from build123d import *

# Parameters (mm, degrees)
BOSS_EXTRUDE1_DEPTH     = 3
SKETCH2_R               = 4
SKETCH2_R_2             = 1.5
BOSS_EXTRUDE2_DEPTH     = 16
BOSS_EXTRUDE4_DEPTH     = 34
SKETCH6_R               = 5
SKETCH6_W               = 13
SKETCH6_H               = 12.705942109
SKETCH6_W_2             = 20
SKETCH6_H_2             = 11.5
CUT_EXTRUDE1_DEPTH      = 10
CUT_EXTRUDE1_DEPTH_BACK = 5
SKETCH9_R               = 12.7
CUT_EXTRUDE3_DEPTH      = 8
SKETCH10_R              = 1
CUT_EXTRUDE4_DEPTH      = 10
FILLET1_R               = 1
SKETCH11_R              = 1.62
SKETCH11_W              = 6.5
SKETCH11_H              = 17.5
CUT_EXTRUDE5_DEPTH      = 10


with BuildPart() as part:
    # Sketch1 → Boss-Extrude1 (new body)
    with BuildSketch(Plane(origin=(0, 0, 0), x_dir=(1, 0, 0), z_dir=(0, 1, 0))):
        with BuildLine():
            Line((-104.6543947, -23.181164953), (-24.598685103, -57.455675883))
            ThreePointArc((-24.598685103, -57.455675883), (62.5, 0), (-24.598685103, 57.455675883))
            Line((-24.598685103, 57.455675883), (-104.6543947, 23.181164953))
            ThreePointArc((-104.6543947, 23.181164953), (-119.94612383, 0), (-104.6543947, -23.181164953))
        make_face()
    extrude(amount=BOSS_EXTRUDE1_DEPTH)

    # Sketch2 → Boss-Extrude2 (add)
    with BuildSketch(Plane(origin=(0, 0, 0), x_dir=(1, 0, 0), z_dir=(0, 1, 0))):
        with Locations((-14.993702206, -24.304194143)):
            Circle(SKETCH2_R)
        with Locations((-14.993702206, -24.304194143)):
            Circle(SKETCH2_R_2, mode=Mode.SUBTRACT)
        with Locations((43.006297794, -24.304194143)):
            Circle(SKETCH2_R)
        with Locations((43.006297794, -24.304194143)):
            Circle(SKETCH2_R_2, mode=Mode.SUBTRACT)
        with Locations((-14.993702206, 24.995805857)):
            Circle(SKETCH2_R)
        with Locations((-14.993702206, 24.995805857)):
            Circle(SKETCH2_R_2, mode=Mode.SUBTRACT)
        with Locations((43.006297794, 24.995805857)):
            Circle(SKETCH2_R)
        with Locations((43.006297794, 24.995805857)):
            Circle(SKETCH2_R_2, mode=Mode.SUBTRACT)
    extrude(amount=BOSS_EXTRUDE2_DEPTH)

    # Sketch3 → Boss-Extrude4 (add)
    with BuildSketch(Plane(origin=(0, 0, 0), x_dir=(1, 0, 0), z_dir=(0, 1, 0))):
        Polygon((-15.993308679, 33.995805857), (-19.886104129, 53.592683168), (-16.090572218, 54.346641522), (-12.643938704, 36.995805857), (43.389376911, 36.995805857), (45.167410352, 33.995805857), align=None)
    extrude(amount=BOSS_EXTRUDE4_DEPTH)

    # Sketch6 → Cut-Extrude1 (cut, two sides)
    with BuildSketch(Plane(origin=(0, 0, -35.995805857), x_dir=(-1, 0, 0), z_dir=(0, 0, -1))) as cut_extrude1_sk:
        with Locations((6.993702206, 21)):
            Circle(SKETCH6_R)
        with Locations((-36.506297794, 20.388898665)):
            Rectangle(SKETCH6_W, SKETCH6_H)
        with Locations((-15.006297794, 21.75)):
            Rectangle(SKETCH6_W_2, SKETCH6_H_2)
    extrude(amount=CUT_EXTRUDE1_DEPTH, mode=Mode.SUBTRACT)
    extrude(cut_extrude1_sk.sketch, amount=-CUT_EXTRUDE1_DEPTH_BACK, mode=Mode.SUBTRACT)

    # Sketch9 → Cut-Extrude3 (cut)
    with BuildSketch(Plane(origin=(0, 3, 0), x_dir=(1, 0, 0), z_dir=(0, 1, 0))):
        with Locations((-19.402851724, 0)):
            Circle(SKETCH9_R)
    extrude(amount=-CUT_EXTRUDE3_DEPTH, mode=Mode.SUBTRACT)

    # Sketch10 → Cut-Extrude4 (cut)
    with BuildSketch(Plane(origin=(0, 3, 0), x_dir=(1, 0, 0), z_dir=(0, 1, 0))):
        with Locations((-116.94612383, 0)):
            Circle(SKETCH10_R)
        with Locations((0, -59.5)):
            Circle(SKETCH10_R)
        with Locations((0, 59.489452719)):
            Circle(SKETCH10_R)
    extrude(amount=-CUT_EXTRUDE4_DEPTH, mode=Mode.SUBTRACT)

    # Fillet1
    fillet1_edges = [part.edges().sort_by_distance(p)[0] for p in [
        (-18.993702206, 3, 24.304194143),
        (39.006297794, 3, 24.304194143),
        (-18.993702206, 3, -24.995805857),
        (39.006297794, 3, -24.995805857),
        (14.587050836, 3, -33.995805857),
        (44.278393631, 3, -35.495805857),
        (15.372719104, 3, -36.995805857),
    ]]
    fillet(fillet1_edges, radius=FILLET1_R)

    # Sketch11 → Cut-Extrude5 (cut)
    with BuildSketch(Plane(origin=(-5.09395257, 0, 1.011881387), x_dir=(-0.19483679, 0, -0.980835677), z_dir=(0.980835677, 0, -0.19483679))):
        with Locations((47.325532424, 29.998886712)):
            Circle(SKETCH11_R)
        with Locations((47.325532424, 14.458886712)):
            Rectangle(SKETCH11_W, SKETCH11_H)
    extrude(amount=-CUT_EXTRUDE5_DEPTH, mode=Mode.SUBTRACT)


solid = part.part
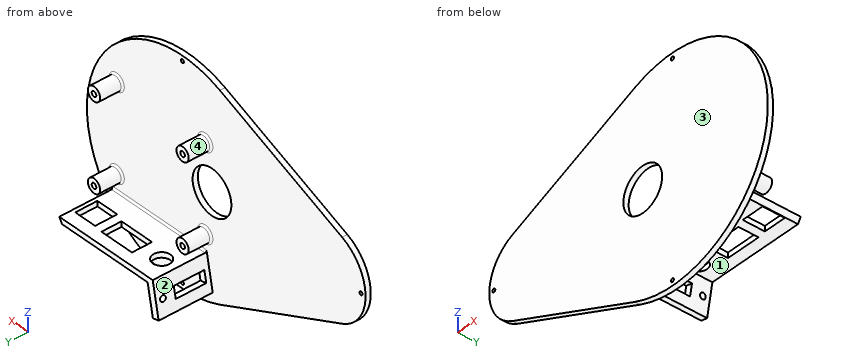
Here's how the part is built. I have some questions about the finished solid (model axes, mm). Face numbers are marked on the shaded views. Round coordinates to 2 decimals unless told otherwise and drop trailing zeros. Loops run counter-clockwise (first coordinate to the right, second up) from the corner with the lowest first, then second, coordinate; pieces in that order, holes last.
1. If we section it at C-C on z = 5: Write out the boundary of the cut face in (x, y).
Answer list:
outline: (-119.45, 0) - (-31.08, 0) - (-31.08, 3) - (-119.45, 3) - close; (-7.73, 0) - (62.3, 0) - (62.3, 3) - (-7.73, 3) - close
2. If we section it at A-A on y = 21: Write out the boundary of the cut face in (x, z), plus the area to 3 significant figures.
Answer list:
outline: (-19.89, -53.59) - (-16.09, -54.35) - (-14.95, -48.59) - (-18.74, -47.84) - close; (-17.48, -41.47) - (-13.68, -42.22) - (-12.64, -37) - (-11.99, -37) - (-11.99, -34) - (-15.99, -34) - close; (-1.99, -37) - (5.01, -37) - (5.01, -34) - (-1.99, -34) - close; (25.01, -37) - (30.01, -37) - (30.01, -34) - (25.01, -34) - close; (43.01, -37) - (43.39, -37) - (45.17, -34) - (43.01, -34) - close
area: 94.5 mm2
3. We'd pull the mould along Z, two halves only. Please class the marked faces 1, 2, 3 and 4: +Z half, -Z half, draft (parallel to the pull), parting line (faces both ways), or undercut.
Answer list:
face 1: -Z half
face 2: undercut
face 3: draft
face 4: undercut
4. If we section it at B-B on x = 16: Write out the boundary of the cut face in (y, z).
Answer list:
outline: (0, -60.42) - (3, -60.42) - (3, -38) arc R1 cw to (4, -37) - (16, -37) - (16, -34) - (4, -34) arc R1 cw to (3, -33) - (3, 60.42) - (0, 60.42) - close; (27.5, -37) - (34, -37) - (34, -34) - (27.5, -34) - close
5. If I drill on line 1 along Z through (x, y) = (0, 1.8); line 2 along Y through (x, z) = (42, 36.5); line 3 along Z through (x, y) = (29.5, 31), over which ranges is the centre line in solid material (lowest first)?
Answer list:
line 1: z = -62.5 to -60.49, -58.49 to 58.5, 60.5 to 62.5
line 2: y = 0 to 3
line 3: z = -37 to -34
6. If we section it at D-D on x = -46: Write out the boundary of the cut face in (y, z), plus the area to 3 significant figures.
Answer list:
outline: (0, -48.29) - (3, -48.29) - (3, 48.29) - (0, 48.29) - close
area: 290 mm2
7. For P1, Ø9, axis at x = 43, z = 24.5, coming from the +Y side; P2, Ø0.9, axis at x = -15.5, z = 24.5, coming from the +Y side; P3, Ø1.5, axis at y = 20.5, z = -36, coming from the -X side; P4, Ø1.8, axis at x = -116.95, z = 0, coming from the +Y side, each with a flat end and sliding along its axis, tell me the tip position at first contact or that it passes through.
Answer list:
P1: stops at y = 16
P2: stops at y = 3
P3: stops at x = -16.54
P4: passes through
